Verification items for the finished model (mm, model axes). Coordinates: 2 decimals unless noted, no trailing zeros. Loops run counter-clockwise (first coordinate to the right, second up) from the corner with the lowest first, then second, coordinate; pieces in that order, holes last.
Q1. Sectioned sample at B-B (x = -238). Enter the section's corners in (y, z).
Q2. Sectioned sample at C-C (z = -268). Enter the section's corners in (x, y).
Q3. Go/stop test with flat-tipped pins: P1, Ø6, axis at y = -7, z = -170, coming from the +X side; P2, Ø9.5, axis at x = 1, y = -2, coming from the -Z side; P3, Ø10, axis at y = 6, z = -301.5, coming from the +X side. Record where each tip stops, or that it passes through.
Q4. Material ranges on probe 1 along X at (y, z) = (-0.5, -235); probe 2 along Z at (x, y) = (-508, 1); probe 3 along X at (y, z) = (4, 22.5), recorded low to high.
Q5. Sectioned sample at A-A (y = 0). Enter the section's corners in (x, z) (3 decimals).
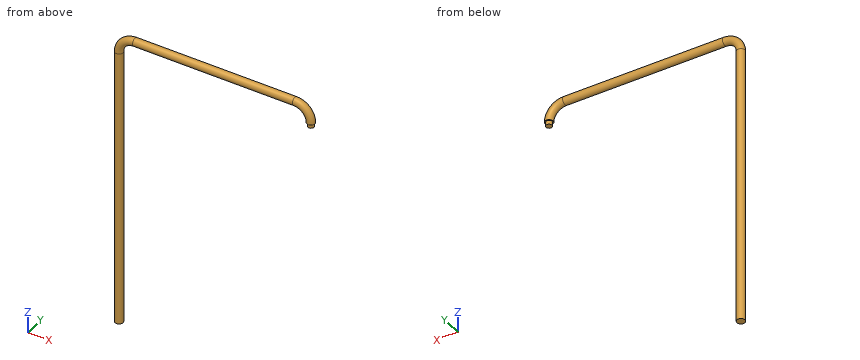
Solid Edge part; units mm, degrees
sketch "Sketch1" plane through (0, 0, 0) normal (0, 0, 1) x (1, 0, 0)
  circle A0 centre (0, 0) radius 9.525
extrude "Protrusion1" add sketch "Sketch1" against normal blind 12.7
sketch "Sketch2" plane through (0, 0, 0) normal (0, -1, 0) x (1, 0, 0)
  arc A0 (0, 0) -> (-50.8, 50.8) centre (-50.8, 0) ccw
  line L0 (-50.8, 50.8) -> (-558.8, 50.8)
  arc A1 (-558.8, 50.8) -> (-609.6, 0) centre (-558.8, 0) ccw
  line L1 (-609.6, 0) -> (-609.6, -889)
sketch "Sketch3" plane through (0, 0, 0) normal (0, 0, 1) x (1, 0, 0)
  circle A0 centre (0, 0) radius 12.7
sweep "SweptProtrusion_1" add profiles "Sketch3" path "Sketch2"
Geometry check:
1. outline: circle Ø25.4 at (0, 50.8)
2. outline: circle Ø25.4 at (-609.6, 0)
3. P1: stops at x = -597.55
3. P2: stops at z = -12.7
3. P3: stops at x = -596.94
4. probe 1: x = -622.29 to -596.91
4. probe 2: z = 38.14 to 63.46
4. probe 3: x = -617.49 to -590.34, -19.26 to 7.89
5. outline: (-622.3, -889) - (-596.9, -889) - (-596.9, 0) arc R38.1 cw to (-558.8, 38.1) - (-50.8, 38.1) arc R38.1 cw to (-12.7, 0) - (-9.525, 0) - (-9.525, -12.7) - (9.525, -12.7) - (9.525, 0) - (12.7, 0) arc R63.5 ccw to (-50.8, 63.5) - (-558.8, 63.5) arc R63.5 ccw to (-622.3, 0) - close
